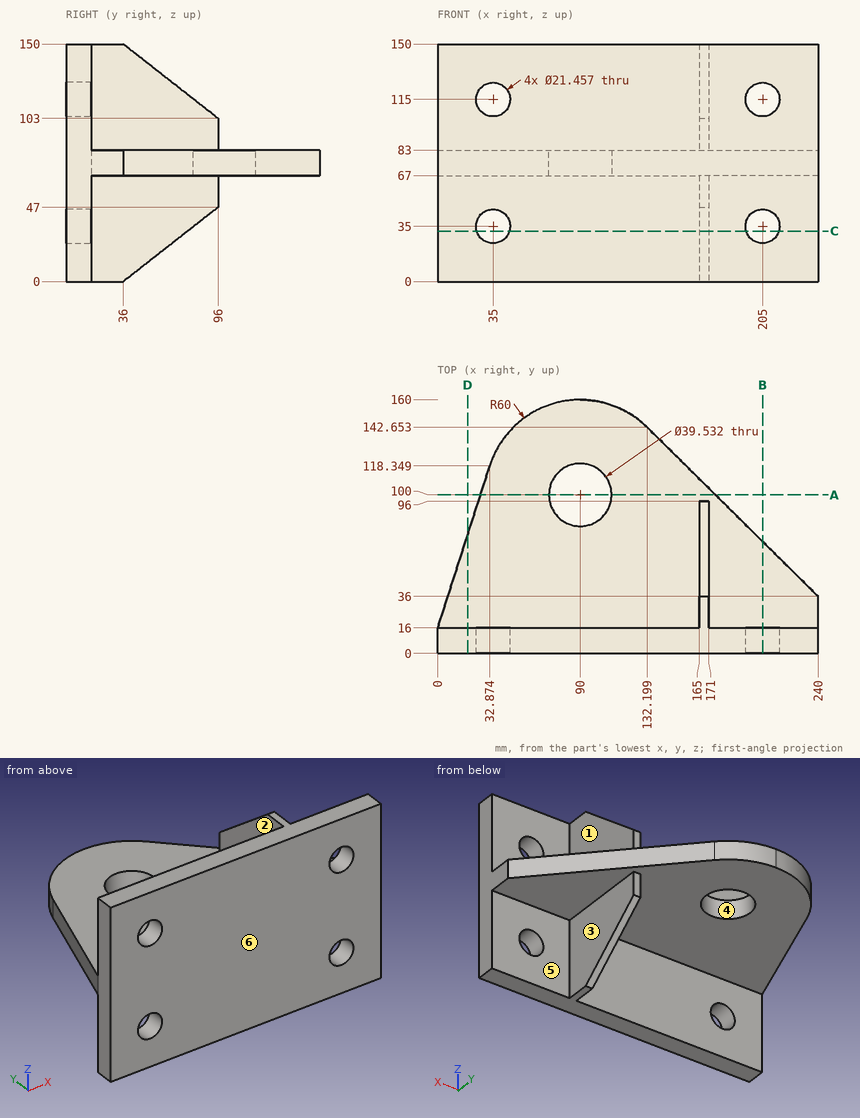
Source: three-view drawing plus pictorial views. Frame: mm from the lowest corner of the part. A direction names the side the tool comes from. Round coordinates to 2 decimals unless told otherwise and drop trailing zeros. Loops run counter-clockwise (first coordinate to the right, second up) from the corner with the lowest first, then second, coordinate; pieces in that order, holes last. Notation, with made-up numbers: (85, -30.5) - (99, -30.5) arc R22 cw to (99, -14.5) - close; hole circle Ø7 at (29, 26.5). An arc over 180 degrees is marked (long way). Write item = value, one per line. Start each with the question number.
Item 1: Mould query, pull axis Y, two halves, no side actions, for the marked faces 4, 5 and 6. Classes: released by +Y, released by -Y, zero draft, split by the parting line, or undercut.
Item 2: Section query D-D on x = 19. Output: boundary loops of the cut face in (y, z), plus the area to 3 significant figures.
Item 3: Material intervals for line 1 (X direction, y = 7, z = 115); line 2 (Z direction, x = 73.5, y = 84); line 3 (Y direction, x = 150, z = 118), sorted ascending.
Item 4: Section query A-A on y = 100. Output: boundary loops of the cut face in (x, z), plus the area to 3 significant figures.
Item 5: First-contact query: pin 1 Ø24.5 at (x, z) = (35, 115) entering from +Y; pin 2 Ø10 at (x, z) = (34.5, 75.5) entering from -Y; pin 3 Ø20 at (y, z) = (41, 26) entering from -X; pin 4 Ø8 at (y, z) = (101.5, 94) entering from -X. Flat tips, straight axial feed; report the tip coordinate or a pass-through.
Item 6: Reachability of the marked faces 1, 2 and 3 from +Z, -Z, +X, -X, +Y, -Y: full face, straight path, thin tool, end or side. Return the list, or none.
Item 7: Section query B-B on x = 205. Output: boundary loops of the cut face in (y, z), plus the area to 3 significant figures.
Item 8: Section query C-C on z = 32. Output: boundary loops of the cut face in (x, y), plus the area to 3 significant figures.
Results list:
q1.face_4 = undercut
q1.face_5 = released by +Y
q1.face_6 = released by -Y
q2.outline = (0, 0) - (16, 0) - (16, 67) - (75.15, 67) - (75.15, 83) - (16, 83) - (16, 150) - (0, 150) - close
q2.area = 3,350 mm²
q3.line_1 = 0 to 24.27, 45.73 to 194.27, 215.73 to 240
q3.line_2 = 67 to 83
q3.line_3 = 0 to 16
q4.outline = (26.98, 67) - (70.23, 67) - (70.23, 83) - (26.98, 83) - close; (109.77, 67) - (175.31, 67) - (175.31, 83) - (109.77, 83) - close
q4.area = 1,740 mm²
q5.pin_1 = 16
q5.pin_2 = 0
q5.pin_3 = 165
q5.pin_4 = through
q6.face_1 = +Z, +X, +Y
q6.face_2 = +Z, -X, +Y
q6.face_3 = -Z, +X, +Y
q7.outline = (0, 0) - (16, 0) - (16, 24.27) - (0, 24.27) - close; (0, 45.73) - (16, 45.73) - (16, 67) - (70.63, 67) - (70.63, 83) - (16, 83) - (16, 104.27) - (0, 104.27) - close; (0, 125.73) - (16, 125.73) - (16, 150) - (0, 150) - close
q7.area = 2,590 mm²
q8.outline = (0, 0) - (24.7, 0) - (24.7, 16) - (0, 16) - close; (45.3, 0) - (194.7, 0) - (194.7, 16) - (171, 16) - (171, 76.85) - (165, 76.85) - (165, 16) - (45.3, 16) - close; (215.3, 0) - (240, 0) - (240, 16) - (215.3, 16) - close
q8.area = 3,550 mm²
